Part print with two shaded views. Sizes in mm from the minimum x, y, z corner. A direction names the side the tool comes from. Round coordinates to 2 decimals unless told otherwise and drop trailing zeros. Order: outer loops, then holes, each group sorted by start corner. A loop starts at its lowest first (then second) coordinate and runs counter-clockwise, first axis right, second up. Notation, with made-up numbers: (-25, 8.5) -> (-11, 8.5) arc R23 cw to (-11, 45.5) -> close; hole circle Ø8 at (65.25, 12). An arc over 180 degrees is marked (long way). Use a Markdown table: item, result. Add a question column.
Item 1: Slice it at A-A, the plane y = 12.7. Give the cut face in (x, z).
Item 2: Pin check, flat tips, straight feed: pin 1 (12 mm diameter, centred on x = 19.5, z = 21, fed in from +Y); pin 2 (12 mm diameter, centred on x = 8, y = 19, fed in from -Z); pin 3 (5 mm diameter, centred on x = 11, z = 6.5, fed in from -Y); pin 4 (2 mm diameter, centred on x = 4.5, z = 26.5, fed in from +Y). Stop position of each tip, or through.
Item 3: Slice it at D-D, the plane z = 28. Give the cut face in (x, y), plus the area to 3 significant figures.
Item 4: 3-axis set-ups, long thin cutter, end or side, ignore diameter. For the marked faces 5 and 6: which of +Z, -Z, +X, -X, +Y, -Y reach the whole face in a straight line?
Item 5: Probe L1, parallel to Y at x = 12.7, z = 16.5; L2, parallel to Z at x = 14, y = 19.5; L3, parallel to Y at x = 11, z = 28.5. List the from-to ranges inside material, lowest first.
Item 6: Slice it at C-C, the plane z = 8.5. Give the cut face in (x, y).
Item 7: Two-plate mould, pull along Z, no slides. Class the marked faces 1, 2, 3 and 4: released by +Z, released by -Z, zero draft, split by the parting line, or undercut.
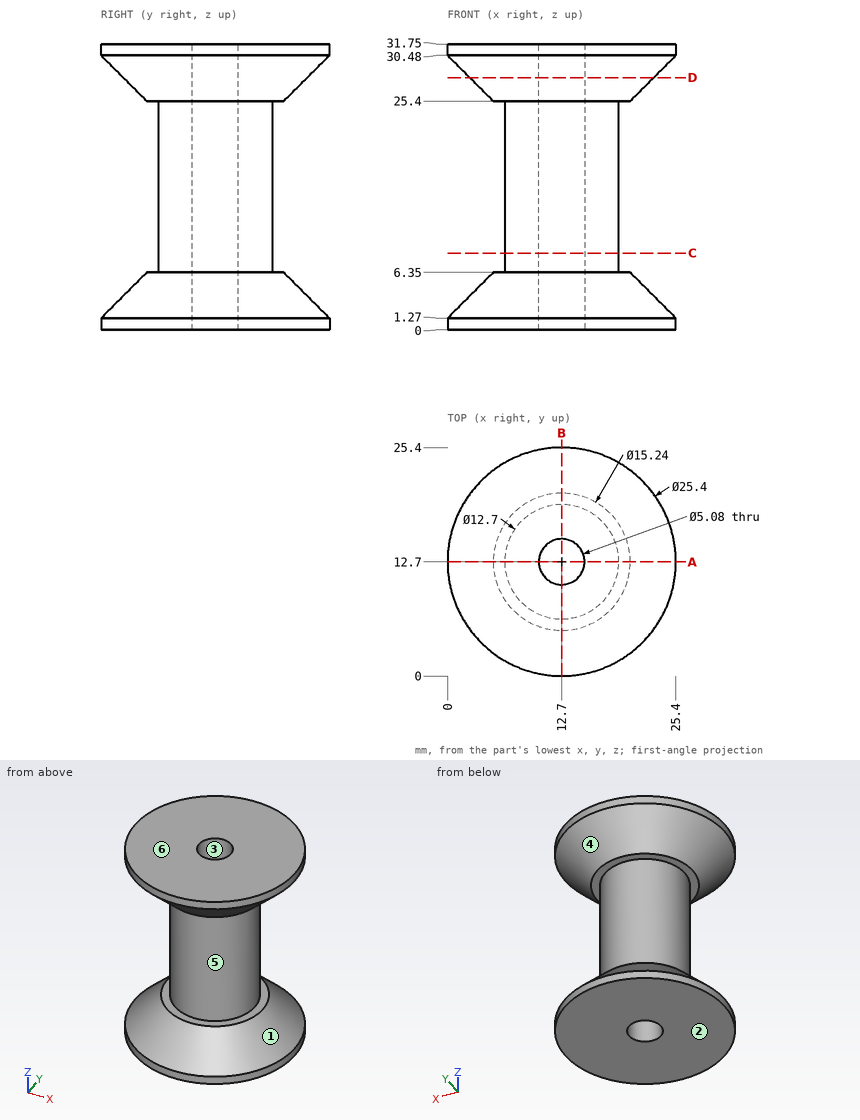
Check sheet entries:
| question | item | result |
|---|---|---|
| 1 | outline | (0, 0) -> (10.16, 0) -> (10.16, 31.75) -> (0, 31.75) -> (0, 30.48) -> (5.08, 25.4) -> (6.35, 25.4) -> (6.35, 6.35) -> (5.08, 6.35) -> (0, 1.27) -> close; (15.24, 0) -> (25.4, 0) -> (25.4, 1.27) -> (20.32, 6.35) -> (19.05, 6.35) -> (19.05, 25.4) -> (20.32, 25.4) -> (25.4, 30.48) -> (25.4, 31.75) -> (15.24, 31.75) -> close |
| 2 | pin 1 | y = 20.24 |
| 2 | pin 2 | z = 0 |
| 2 | pin 3 | y = 2.85 |
| 2 | pin 4 | y = 18.43 |
| 3 | outline | circle Ø20.44 at (12.7, 12.7); hole circle Ø5.08 at (12.7, 12.7) |
| 3 | area | 308 mm2 |
| 4 | face 5 | none |
| 4 | face 6 | +Z, +X, -X, +Y, -Y |
| 5 | L1 | 6.35 to 10.16, 15.24 to 19.05 |
| 5 | L2 | 0 to 6.35, 25.4 to 31.75 |
| 5 | L3 | 2.12 to 10.81, 14.59 to 23.28 |
| 6 | outline | circle Ø12.7 at (12.7, 12.7); hole circle Ø5.08 at (12.7, 12.7) |
| 7 | face 1 | undercut |
| 7 | face 2 | released by -Z |
| 7 | face 3 | zero draft |
| 7 | face 4 | undercut |
